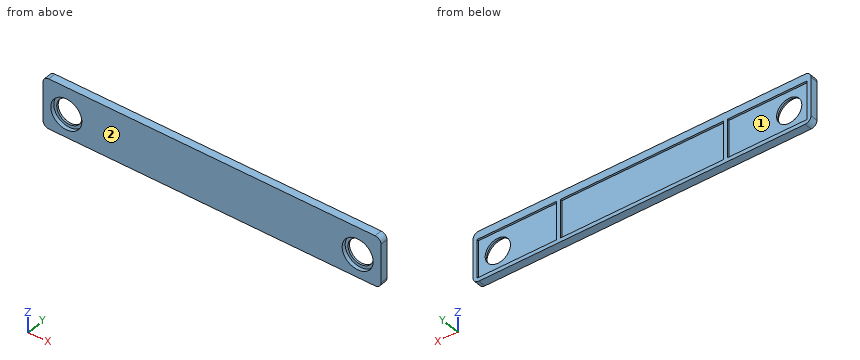
Autodesk Inventor part; units mm, degrees
ref_plane "YZ Plane" through (0, 0, 0) normal (1, 0, 0) x (0, 1, 0)
ref_plane "XZ Plane" through (0, 0, 0) normal (0, 1, 0) x (-1, 0, 0)
ref_plane "XY Plane" through (0, 0, 0) normal (0, 0, 1) x (1, 0, 0)
sketch "Sketch1" plane through (0, 0, 0) normal (0, 1, 0) x (-1, 0, 0)
  line L0 (172, 20) -> (172, 0)
  line L1 (2, 20) -> (2, 0)
  line L2 (43, 20) -> (43, 0)
  line L3 (131, 20) -> (131, 0)
  line L4 (129, 20) -> (129, 0)
  line L5 (174, 24) -> (174, 0)
  line L6 (45, 20) -> (45, 0)
  line L7 (0, 24) -> (0, 0)
  line L8 (0, 0) -> (174, 0)
  line L9 (0, 24) -> (174, 24)
  line L10 (131, 20) -> (172, 20)
  line L11 (2, 20) -> (43, 20)
  line L12 (45, 20) -> (129, 20)
  line L13 (0, 0) -> (174, 0)
  line L14 (174, 0) -> (174, -2)
  line L15 (174, -2) -> (0, -2)
  line L16 (0, -2) -> (0, 0)
  line L17 (2, 10) -> (172, 10) construction
  line L18 (162, 20) -> (162, 0) construction
  line L19 (12, 20) -> (12, 0) construction
  circle A0 centre (12, 10) radius 8
  circle A1 centre (12, 10) radius 6.5
  circle A2 centre (162, 10) radius 6.5
  circle A3 centre (162, 10) radius 8
  dimension "d4" = 41
  dimension "d5" = 41
  dimension "d7" = 2
  dimension "d8" = 2
  dimension "d9" = 2
  dimension "d10" = 2
  dimension "d12" = 174
  dimension "d17" = 4
  dimension "d20" = 20
  dimension "d21" = 2
  dimension "d22" = 10
  dimension "d23" = 10
  dimension "d24" = 16
  dimension "d25" = 13
extrude "Extrusion1" add sketch "Sketch1" against normal blind 3 contours L10 L3 L8 L4 L12 L6 L2 L11 L1 L7 L9 L5 L0 | L0 L8 L3 L10 | L8 L14 L15 L16 | L8 L6 L12 L4 | L8 L1 L11 L2
extrude "Extrusion2" add sketch "Sketch1" along normal blind 1 contours L10 L3 L8 L4 L12 L6 L2 L11 L1 L7 L9 L5 L0 | L8 L14 L15 L16
extrude "Extrusion3" add sketch "Sketch1" against normal blind 1 contours A0 | A3
fillet "Fillet1" radius 3 4 edges at (-174, -1, -2) (-174, -1, 24) (0, -1, 24) (0, -1, -2)
properties part number "arm1a"
The listing builds one solid part. Answer for the finished solid, in the listing's coordinates (mm). Face numbers are marked on the shaded views. Coordinates: 2 decimals unless noted, no trailing zeros. Write each loop counter-clockwise with the first axis right and the second up, starting at its lowest first coordinate (ties: lowest second). Pieces come first, ordered by that corner, then holes. Notation, with made-up numbers: M -23.75,-13.5 L -17.75,-13.5 A23 cw -17.75,3.5 Z; hole C 89,-3.5 d4. An arc over 180 degrees is marked long. Put each result on its own line as item: value. Start each with the question number.
1. Flat-ended cylindrical pins translate along their axes: P1, Ø14.5, axis at x = -12, z = 10, coming from the -Y side; P2, Ø6, axis at x = -115, z = 9.5, coming from the +Y side; P3, Ø10.5, axis at x = -162, z = 10, coming from the -Y side. Find the tip coordinate at first contact, or state that the pin passes through.
2. Consider line 1 (X direction, y = -2.35, z = 10.75); line 2 (Z direction, x = -162, y = -1.9); line 3 (Z direction, x = -115, y = 0.5). Determine where each line is inside the solid, lowest interval first. Write a range as from..to.
3. A cutting plane is placed at D-D on x = -135. Write down the section's boundary in (y, z), then the cut area to 3 significant figures.
4. A cutting plane is placed at A-A on z = 10. Count the separate pieces of the cut face and the enclosed holes in it, then the cut area to 3 significant figures.
5. A cutting plane is placed at C-C on y = -2. Write down the section's boundary in (x, z).
6. A cutting plane is placed at B-B on x = -12. Write down the section's boundary in (y, z), then the cut area to 3 significant figures.
7. For a pull along Z with two mould halves and no side action, classify the marked faces 1 and 2 as pulls with the +Z half, pulls with the -Z half, needs draft (parallel to the pull), parting line crosses it, or undercut.
Resolved:
1. P1: stops at y = -1
1. P2: stops at y = 0
1. P3: passes through
2. line 1: x = -174..-169.96, -154.04..-19.96, -4.04..0
2. line 2: z = -2..2, 18..24
2. line 3: z = -2..0, 20..24
3. outline: M -3,-2 L 1,-2 L 1,0 L 0,0 L 0,20 L 1,20 L 1,24 L -3,24 Z
3. area: 84.0 mm2
4. separate pieces: 3
4. enclosed holes: 0
4. area: 440 mm2
5. outline: M -174,1 A3 ccw -171,-2 L -3,-2 A3 ccw 0,1 L 0,21 A3 ccw -3,24 L -171,24 A3 ccw -174,21 Z; hole C -162,10 d16; hole C -12,10 d16
6. outline: M -3,-2 L 1,-2 L 1,0 L 0,0 L 0,3.5 L -1,3.5 L -1,2 L -3,2 Z; M -3,18 L -1,18 L -1,16.5 L 0,16.5 L 0,20 L 1,20 L 1,24 L -3,24 Z
6. area: 39.0 mm2
7. face 1: undercut
7. face 2: needs draft
